The drawing under review shows one solid part. Ordinate dimensions are in mm from its lowest x, y, z. Give positions to 0.01 mm unless a question says otherwise; leave off trailing zeros. Write each loop counter-clockwise with the first axis right and the second up, starting at its lowest first coordinate (ties: lowest second). Pieces come first, ordered by that corner, then holes. Notation, with made-up numbers: (47.25, 88.25) -> (74.25, 88.25) arc R17 cw to (74.25, 96.25) -> close; hole circle Ø8 at (75.25, 56). An arc over 180 degrees is marked (long way). Use CSV: the item, a comma, the result in double quotes.
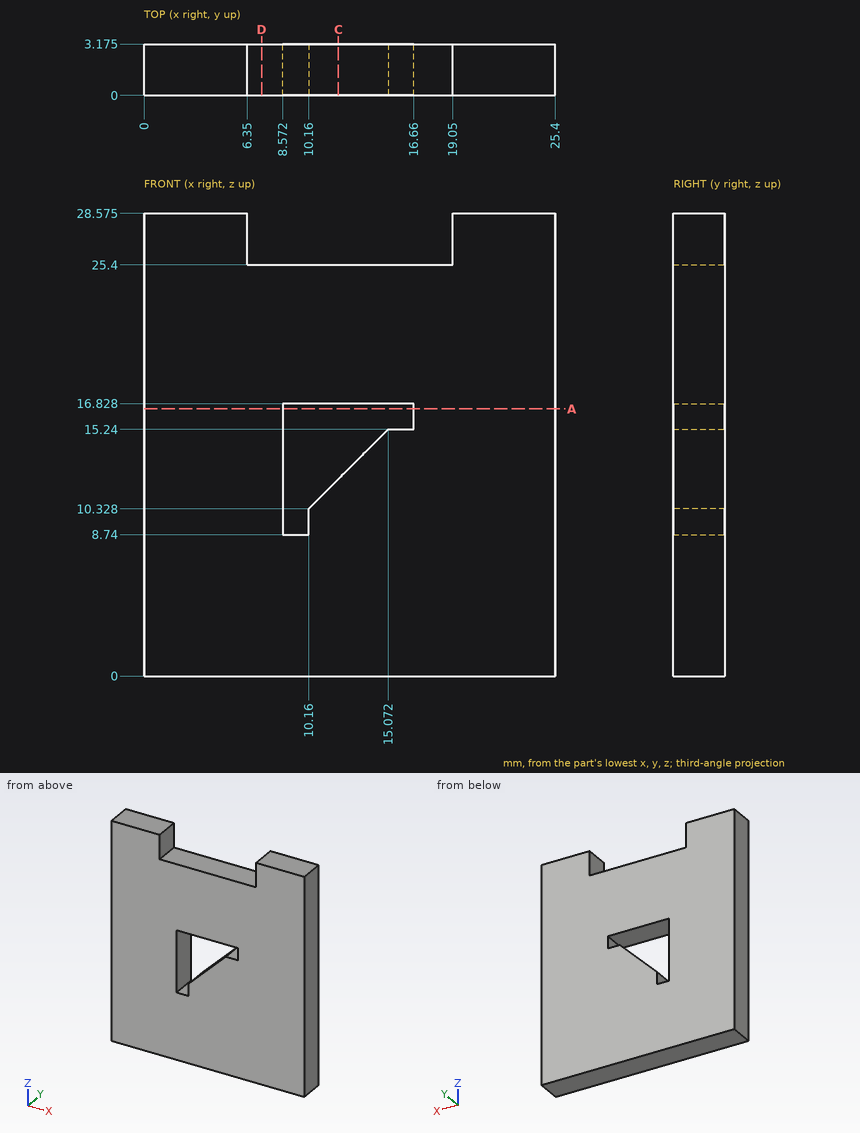
(1) Clearance check with flat-ended pins moving along their axes: pin 1 (4 mm diameter, centred on x = 11, z = 11.5, fed in from +Y) (1 decimal); pin 2 (1 mm diameter, centred on x = 12.5, y = 1, fed in from +Z). State where each tip first meets the part, or that it passes through.
Established:
pin 1,"stops at y = 3.2"
pin 2,"stops at z = 25.4"
(2) Take a section at D-D (x = 7.25). Write out the cut boundary in (y, z) (1 decimal).
Established:
outline,"(0, 0) -> (3.2, 0) -> (3.2, 25.4) -> (0, 25.4) -> close"
(3) For line 1 along X through (y, z) = (2.7, 15.5); line 2 along Z through (x, y) = (16.5, 0.8); line 3 along X through (y, z) = (0.25, 9.25), list the stretches that pass through material, from the lowest coordinate up. Write a range as [from, to].
Established:
line 1,"x = [0, 8.57], [16.66, 25.4]"
line 2,"z = [0, 15.24], [16.83, 25.4]"
line 3,"x = [0, 8.57], [10.16, 25.4]"
(4) Take a section at C-C (x = 12). Write out the cut boundary in (y, z) (1 decimal).
Established:
outline,"(0, 0) -> (3.2, 0) -> (3.2, 12.2) -> (0, 12.2) -> close; (0, 16.8) -> (3.2, 16.8) -> (3.2, 25.4) -> (0, 25.4) -> close"
(5) Take a section at A-A (z = 16.5). Write out the cut boundary in (x, y) (1 decimal).
Established:
outline,"(0, 0) -> (8.6, 0) -> (8.6, 3.2) -> (0, 3.2) -> close; (16.7, 0) -> (25.4, 0) -> (25.4, 3.2) -> (16.7, 3.2) -> close"
